```python
from build123d import *

# Parameters (mm, degrees)
SKETCH_1_W             = 42
SKETCH_1_H             = 42
EXTRUDE_1_DEPTH        = 60
CHAMFER_1_SIZE         = 5
CUT_EXTRUDE_1_DEPTH    = 43
EXTRUDE_2_DEPTH        = 11
SKETCH_4_R             = 21
EXTRUDE_3_DEPTH        = 49.2
SKETCH_5_W             = 56
SKETCH_5_H             = 42
EXTRUDE_4_DEPTH        = 42
CHAMFER_2_SIZE         = 1
HOLE_WIZARD_M4_1_D     = 3.3
HOLE_WIZARD_M4_1_DEPTH = 10.1
HOLE_WIZARD_M4_1_TIP   = 0.991420021
SKETCH_10_R            = 11
EXTRUDE_5_DEPTH        = 2
SKETCH_11_R            = 4
EXTRUDE_6_DEPTH        = 20
CHAMFER_3_SIZE         = 0.5
EXTRUDE_7_DEPTH        = 1.2
EXTRUDE_7_DEPTH_BACK   = 1


with BuildPart() as part:
    # 스케치1 → 보스-돌출1 (new body)
    with BuildSketch(Plane.XY):
        Rectangle(SKETCH_1_W, SKETCH_1_H)
    extrude(amount=EXTRUDE_1_DEPTH)

    # 모따기1
    chamfer_1_edges = [part.edges().sort_by_distance(p)[0] for p in [
        (21, 21, 30),
        (21, -21, 30),
        (-21, 21, 30),
        (-21, -21, 30),
        (-21, 21, 30),
        (-21, -21, 30),
        (21, 21, 30),
        (21, -21, 30),
        (21, -21, 30),
        (-21, -21, 30),
        (-21, 21, 30),
        (21, 21, 30),
    ]]
    chamfer(chamfer_1_edges, length=CHAMFER_1_SIZE)

    # 스케치2 → 컷-돌출1 (cut)
    with BuildSketch(Plane.XY.offset(51)):
        Polygon((-11, 21), (-21, 21), (-21, 11), align=None)
        Polygon((21, 11), (21, 21), (11, 21), align=None)
        Polygon((11, -21), (21, -21), (21, -11), align=None)
        Polygon((-21, -11), (-21, -21), (-11, -21), align=None)
    extrude(amount=-CUT_EXTRUDE_1_DEPTH, mode=Mode.SUBTRACT)

    # 스케치3 → 보스-돌출2 (add)
    with BuildSketch(Plane(origin=(0, 0, 0), x_dir=(-1, 0, 0), z_dir=(0, 0, -1))):
        Polygon((-16, 21), (-21, 16), (-21, -16), (-16, -21), (16, -21), (21, -16), (21, 16), (16, 21), align=None)
    extrude(amount=EXTRUDE_2_DEPTH)

    # 스케치4 → 보스-돌출3 (add)
    with BuildSketch(Plane(origin=(0, 0, -11), x_dir=(-1, 0, 0), z_dir=(0, 0, -1))):
        Circle(SKETCH_4_R)
    extrude(amount=EXTRUDE_3_DEPTH)

    # 스케치5 → 보스-돌출4 (add)
    with BuildSketch(Plane(origin=(0, 0, -60.2), x_dir=(-1, 0, 0), z_dir=(0, 0, -1))):
        Rectangle(SKETCH_5_W, SKETCH_5_H)
    extrude(amount=EXTRUDE_4_DEPTH)

    # 모따기2
    # the kernel refuses this chamfer: 1 mm, written as the material it takes off along each edge
    with BuildSketch(Plane(origin=(-27.333333333, 20.333333333, -60.866666667), x_dir=(0.7071067811865475, 0.7071067811865475, 0), z_dir=(-0.5773502691896258, 0.5773502691896258, 0.5773502691896258)), Plane(origin=(-27.333333333, -20.333333333, -60.866666667), x_dir=(-0.7071067811865475, 0.7071067811865475, 0), z_dir=(-0.5773502691896258, -0.5773502691896258, 0.5773502691896258)), Plane(origin=(27.333333333, 20.333333333, -60.866666667), x_dir=(0.7071067811865475, -0.7071067811865475, 0), z_dir=(0.5773502691896258, 0.5773502691896258, 0.5773502691896258)), Plane(origin=(27.333333333, -20.333333333, -101.533333333), x_dir=(0.7071067811865475, 0.7071067811865475, 0), z_dir=(0.5773502691896258, -0.5773502691896258, -0.5773502691896258))) as chamfer_2_piece_1:
        Polygon((-0.707106781, 0.40824829), (0.707106781, 0.40824829), (0, -0.816496581), align=None)
    extrude(amount=1.270170592, mode=Mode.SUBTRACT)
    with BuildSketch(Plane(origin=(-27.333333333, -20.333333333, -101.533333333), x_dir=(-0.7071067811865475, 0.7071067811865475, 0), z_dir=(-0.5773502691896258, -0.5773502691896258, -0.5773502691896258)), Plane(origin=(-27.333333333, 20.333333333, -101.533333333), x_dir=(0.7071067811865475, 0.7071067811865475, 0), z_dir=(-0.5773502691896258, 0.5773502691896258, -0.5773502691896258)), Plane(origin=(27.333333333, -20.333333333, -60.866666667), x_dir=(0.7071067811865475, 0.7071067811865475, 0), z_dir=(0.5773502691896258, -0.5773502691896258, 0.5773502691896258)), Plane(origin=(27.333333333, 20.333333333, -101.533333333), x_dir=(0.7071067811865475, -0.7071067811865475, 0), z_dir=(0.5773502691896258, 0.5773502691896258, -0.5773502691896258))) as chamfer_2_piece_2:
        Polygon((-0.707106781, -0.40824829), (0.707106781, -0.40824829), (0, 0.816496581), align=None)
    extrude(amount=1.270170592, mode=Mode.SUBTRACT)
    with BuildSketch(Plane(origin=(-28, 23.571682988, -60.2), x_dir=(0.9996219169112968, 0, 0.0274958766105891), z_dir=(0, -1, 0)), Plane(origin=(-28, -21, -57.628317012), x_dir=(0.9996219169112968, -0.027495876610585647, 0), z_dir=(0, 0, -1)), Plane(origin=(-28, 21, -57.628317012), x_dir=(-0.027495876610585647, -0.9996219169112968, 0), z_dir=(0, 0, -1)), Plane(origin=(28, -23.571682988, -60.2), x_dir=(-0.9996219169112968, 0, 0.0274958766105891), z_dir=(0, 1, 0)), Plane(origin=(28, 21, -57.628317012), x_dir=(-0.9996219169112968, 0.027495876610585647, 0), z_dir=(0, 0, -1)), Plane(origin=(-28, 23.571682988, -102.2), x_dir=(-0.02749587661058574, 0, 0.9996219169112968), z_dir=(0, -1, 0)), Plane(origin=(28, -23.571682988, -102.2), x_dir=(0.02749587661058574, 0, 0.9996219169112968), z_dir=(0, 1, 0))) as chamfer_2_piece_3:
        Polygon((CHAMFER_2_SIZE * 0.999621916911, -CHAMFER_2_SIZE * 0.0274958766106), (-CHAMFER_2_SIZE * 0.0274958766106, -CHAMFER_2_SIZE * 0.999621916911), (0, 0), align=None)
    extrude(amount=47.143365976, mode=Mode.SUBTRACT)
    with BuildSketch(Plane(origin=(0, 21, -60.2), x_dir=(0, -0.9996219169112968, 0.0274958766105891), z_dir=(-1, 0, 0))) as chamfer_2_piece_4_section:
        Polygon((CHAMFER_2_SIZE * 0.999621916911, -CHAMFER_2_SIZE * 0.0274958766106), (-CHAMFER_2_SIZE * 0.0274958766106, -CHAMFER_2_SIZE * 0.999621916911), (0, 0), align=None)
    chamfer_2_piece_4 = extrude(amount=30.571682988, mode=Mode.PRIVATE)
    chamfer_2_piece_4 = chamfer_2_piece_4 - Plane(origin=(0, 0, -60.539954397), x_dir=(-1, 0, 0), z_dir=(0, 0, 1)) * Cylinder(21, 66, mode=Mode.PRIVATE)
    add(chamfer_2_piece_4, mode=Mode.SUBTRACT)
    with BuildSketch(Plane(origin=(30.571682988, 21, -60.2), x_dir=(0, -0.9996219169112968, 0.0274958766105891), z_dir=(-1, 0, 0))) as chamfer_2_piece_5_section:
        Polygon((CHAMFER_2_SIZE * 0.999621916911, -CHAMFER_2_SIZE * 0.0274958766106), (-CHAMFER_2_SIZE * 0.0274958766106, -CHAMFER_2_SIZE * 0.999621916911), (0, 0), align=None)
    chamfer_2_piece_5 = extrude(amount=30.571682988, mode=Mode.PRIVATE)
    chamfer_2_piece_5 = chamfer_2_piece_5 - Plane(origin=(0, 0, -60.539954397), x_dir=(-1, 0, 0), z_dir=(0, 0, 1)) * Cylinder(21, 66, mode=Mode.PRIVATE)
    add(chamfer_2_piece_5, mode=Mode.SUBTRACT)
    with BuildSketch(Plane(origin=(4.1e-08, -21, -60.2), x_dir=(0, 0.9996219169112968, 0.0274958766105891), z_dir=(1, 0, 0))) as chamfer_2_piece_6_section:
        Polygon((CHAMFER_2_SIZE * 0.999621916911, -CHAMFER_2_SIZE * 0.0274958766106), (-CHAMFER_2_SIZE * 0.0274958766106, -CHAMFER_2_SIZE * 0.999621916911), (0, 0), align=None)
    chamfer_2_piece_6 = extrude(amount=30.571682947, mode=Mode.PRIVATE)
    chamfer_2_piece_6 = chamfer_2_piece_6 - Plane(origin=(0, 0, -60.539954397), x_dir=(-1, 0, 0), z_dir=(0, 0, 1)) * Cylinder(21, 66, mode=Mode.PRIVATE)
    add(chamfer_2_piece_6, mode=Mode.SUBTRACT)
    with BuildSketch(Plane(origin=(-30.571682988, -21, -60.2), x_dir=(0, 0.9996219169112968, 0.0274958766105891), z_dir=(1, 0, 0))) as chamfer_2_piece_7_section:
        Polygon((CHAMFER_2_SIZE * 0.999621916911, -CHAMFER_2_SIZE * 0.0274958766106), (-CHAMFER_2_SIZE * 0.0274958766106, -CHAMFER_2_SIZE * 0.999621916911), (0, 0), align=None)
    chamfer_2_piece_7 = extrude(amount=30.571683029, mode=Mode.PRIVATE)
    chamfer_2_piece_7 = chamfer_2_piece_7 - Plane(origin=(0, 0, -60.539954397), x_dir=(-1, 0, 0), z_dir=(0, 0, 1)) * Cylinder(21, 66, mode=Mode.PRIVATE)
    add(chamfer_2_piece_7, mode=Mode.SUBTRACT)
    with BuildSketch(Plane(origin=(28, -21, -57.628317012), x_dir=(-0.9996219169112968, -0.027495876610585647, 0), z_dir=(0, 0, -1))) as chamfer_2_piece_8:
        Polygon((CHAMFER_2_SIZE * 0.999621916911, CHAMFER_2_SIZE * 0.0274958766106), (-CHAMFER_2_SIZE * 0.0274958766106, CHAMFER_2_SIZE * 0.999621916911), (0, 0), align=None)
    extrude(amount=47.143365976, mode=Mode.SUBTRACT)
    with BuildSketch(Plane(origin=(30.571682988, 21, -102.2), x_dir=(0, 0.02749587661058574, 0.9996219169112968), z_dir=(-1, 0, 0)), Plane(origin=(-30.571682988, -21, -102.2), x_dir=(0, -0.02749587661058574, 0.9996219169112968), z_dir=(1, 0, 0))) as chamfer_2_piece_9:
        Polygon((CHAMFER_2_SIZE * 0.999621916911, -CHAMFER_2_SIZE * 0.0274958766106), (-CHAMFER_2_SIZE * 0.0274958766106, -CHAMFER_2_SIZE * 0.999621916911), (0, 0), align=None)
    extrude(amount=61.143365976, mode=Mode.SUBTRACT)

    # M4 나사 구멍1
    with Locations(Plane.ZY.offset(28)):
        with Locations((-96.074368671, 12.374368671), (-71.325631329, 12.374368671), (-71.325631329, -12.374368671), (-96.074368671, -12.374368671)):
            Hole(HOLE_WIZARD_M4_1_D / 2, depth=HOLE_WIZARD_M4_1_DEPTH)
            with Locations((0, 0, -(HOLE_WIZARD_M4_1_DEPTH + HOLE_WIZARD_M4_1_TIP / 2))):  # 118° drill point
                Cone(0, HOLE_WIZARD_M4_1_D / 2, HOLE_WIZARD_M4_1_TIP, mode=Mode.SUBTRACT)

    # 스케치10 → 보스-돌출5 (add)
    with BuildSketch(Plane.ZY.offset(28)):
        with Locations(Location((-83.7, 0, 0), (0, 0, 90))):
            Circle(SKETCH_10_R)
    extrude(amount=EXTRUDE_5_DEPTH)

    # 스케치11 → 보스-돌출6 (add)
    with BuildSketch(Plane.ZY.offset(30)):
        with Locations(Location((-83.7, 0, 0), (0, 0, 270))):
            Circle(SKETCH_11_R)
    extrude(amount=EXTRUDE_6_DEPTH)

    # 모따기3
    chamfer_3_edges = [part.edges().sort_by_distance(p)[0] for p in [
        (-50, 4, -83.7),
    ]]
    chamfer(chamfer_3_edges, length=CHAMFER_3_SIZE)

    # 스케치12 → 보스-돌출7 (add, two sides: drawn at the far end of the back side and taken through both)
    with BuildSketch(Plane(origin=(0, 0, -87.7), x_dir=(-1, 0, 0), z_dir=(0, 0, -1)).offset(-EXTRUDE_7_DEPTH_BACK)):
        with BuildLine():
            Line((37.5, 2), (44.5, 2))
            ThreePointArc((44.5, 2), (46.5, 0), (44.5, -2))
            Line((44.5, -2), (37.5, -2))
            ThreePointArc((37.5, -2), (35.5, 0), (37.5, 2))
        make_face()
    extrude(amount=EXTRUDE_7_DEPTH + EXTRUDE_7_DEPTH_BACK)


solid = part.part
```
The model under review builds one solid part; all positions refer to its coordinate system, in mm. A direction names the side the tool comes from. Round coordinates to 2 decimals unless told otherwise and drop trailing zeros. Write each loop counter-clockwise with the first axis right and the second up, starting at its lowest first coordinate (ties: lowest second). Pieces come first, ordered by that corner, then holes. Notation, with made-up numbers: M 2.5,42 L 7.5,42 A13 cw 7.5,49 Z; hole C -3.5,66.25 d4. An arc over 180 degrees is marked long. Use CSV: the item, a comma, the result in double quotes. Start each with the question number.
(1) Clearance check with flat-ended pins moving along their axes: P1, Ø3, axis at y = 12.37, z = -71.33, coming from the -X side; P2, Ø10, axis at y = -15.5, z = 41, coming from the +X side; P3, Ø2, axis at y = -6.5, z = -46.5, coming from the -X side. State where each tip first meets the part, or that it passes through.
(2) We need section C-C, the plane y = 6. State the section outline as (x, z) points, then the cut area to 3 significant figures.
(3) We need section D-D, the plane z = -83.7. State the section outline as (x, y) points.
(4) Tool access review of faces 4 (the face through (18, 19, -1)), 5 (the face through (21.4, 0.3, -60.2)), 6 (the face through (16, -16, 30)), 7 (the face through (-17, 17, 51)), 8 (the face through (-22.88, 12.87, -72.9)): name each direction out of +Z, -Z, +X, -X, +Y, -Y from which nothing blocks a thin tool from reaching the whole face with its end or side.
(5) We need section B-B, the plane x = -34. State the section outline as (y, z) points, then the cut area to 3 significant figures.
(6) For line 1 along Z through (x, y) = (19.5, 11); line 2 along X through (y, z) = (-11.5, -82); line 3 along Z through (x, y) = (22, 9), list the stretches that pass through material, from the lowest coordinate up.
(7) The part is to be moulded in two halves that separate along Y. For faces 1 (the face through (-16, 16, 30)), 2 (the face through (-17.08, -12.29, -95.8)), 3 (the face through (16, 15, -11)), say which applies: +Y half, -Y half, draft (parallel to the pull), parting line (faces both ways), or undercut.
(8) We need section A-A, the plane z = -1. State the section outline as (x, y) points, then the cut area to 3 significant figures.
Findings:
1,P1,"x = -17.81"
1,P2,"x = 21"
1,P3,"x = -20.27"
2,outline,"M -30,-92.92 L -28,-92.92 L -28,-101.2 L -27,-102.2 L 27,-102.2 L 28,-101.2 L 28,-61.2 L 27,-60.2 L 20.12,-60.2 L 20.12,-11 L 21,-11 L 21,60 L -21,60 L -21,-11 L -20.12,-11 L -20.12,-60.2 L -27,-60.2 L -28,-61.2 L -28,-74.48 L -30,-74.48 Z"
2,area,"7,350 mm^2"
3,outline,"M -50,-3.5 L -49.5,-4 L -30,-4 L -30,-11 L -28,-11 L -28,-20 L -27,-21 L 27,-21 L 28,-20 L 28,20 L 27,21 L -27,21 L -28,20 L -28,11 L -30,11 L -30,4 L -49.5,4 L -50,3.5 Z"
4,face 4,"+Z, +X, +Y"
4,face 5,"+X"
4,face 6,"+X, -Y"
4,face 7,"-X, +Y"
4,face 8,"-X"
5,outline,"C 0,-83.7 d8"
5,area,"50.3 mm^2"
6,line 1,"-102.2 to -60.2, -11 to 60"
6,line 2,"-28 to 28"
6,line 3,"-102.2 to -60.2"
7,face 1,"+Y half"
7,face 2,"undercut"
7,face 3,"draft"
8,outline,"M -21,-16 L -16,-21 L 16,-21 L 21,-16 L 21,16 L 16,21 L -16,21 L -21,16 Z"
8,area,"1,710 mm^2"
